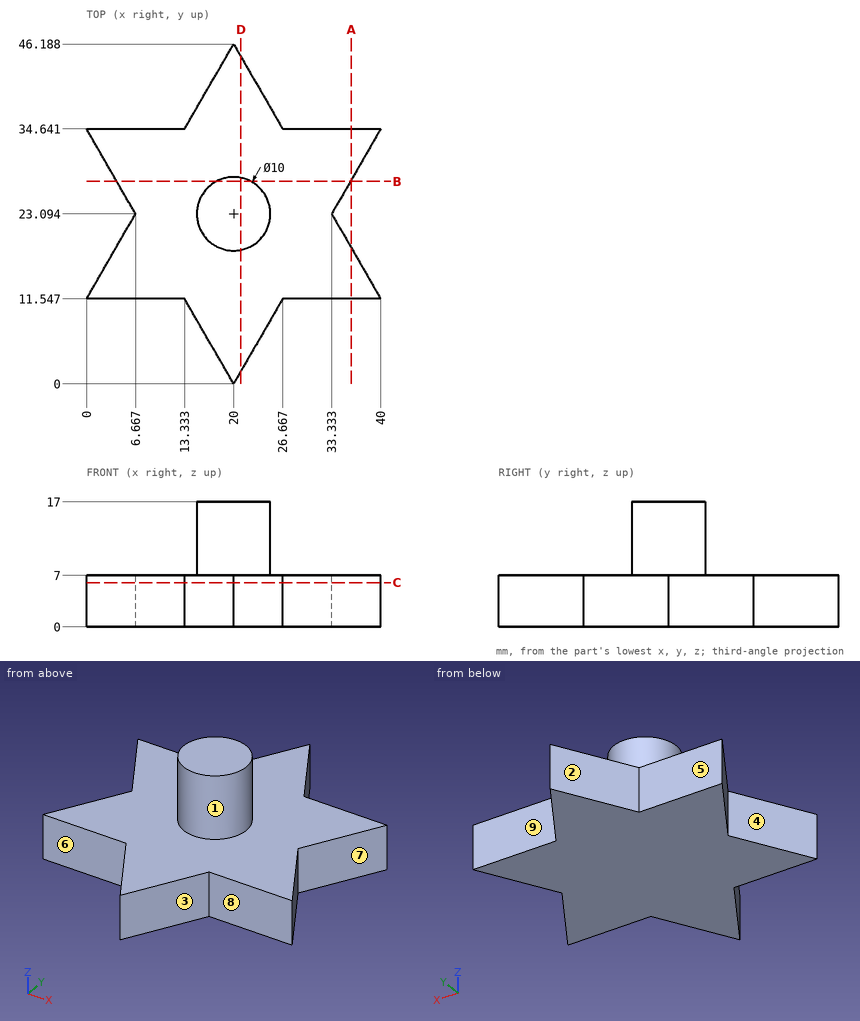
Drawing for the job (mm, zero at the part's lowest x, y, z). A direction names the side the tool comes from. Give positions to 0.01 mm unless a question says otherwise; leave off trailing zeros. Loops run counter-clockwise (first coordinate to the right, second up) from the corner with the lowest first, then second, coordinate; pieces in that order, holes last. Notation, with made-up numbers: M 7.25,-11.5 L 40.25,-11.5 A13 cw 40.25,2.5 Z; hole C 34,29 d5. An arc over 180 degrees is marked long. Use one line per item in the form item = value.
Item 1: Flat gauge pins, fed straight in: pin 1 (1.5 mm diameter, centred on x = 28.5, z = 5.5, fed in from +Y); pin 2 (1 mm diameter, centred on x = 24.5, z = 12.5, fed in from -Y) (1 decimal); pin 3 (8 mm diameter, centred on y = 19, z = 8, fed in from +X); pin 4 (8 mm diameter, centred on x = 4.5, y = 28, fed in from -Z). Where does each tip first touch, or does it go through?
Determined:
pin_1 = 34.64
pin_2 = 20.1
pin_3 = 37.93
pin_4 = 0
Item 2: Which spindle directions (+Z, -Z, +X, -X, +Y, -Y) get a long thin tool onto all of the face, cutting with end or side? Do the marked faces 5, 6, 7, 8 and 9. Say none if no direction does.
Determined:
face_5 = +Z, -Z, -X, +Y
face_6 = +Z, -Z, -X, -Y
face_7 = +Z, -Z, +X
face_8 = +Z, -Z, +X, -Y
face_9 = +Z, -Z, +X, +Y
Item 3: Slice it at A-A (x = 36). List the corners of the cut face in (y, z) (1 decimal), plus the area to 3 significant figures.
Determined:
outline = M 11.5,0 L 18.5,0 L 18.5,7 L 11.5,7 Z; M 27.7,0 L 34.6,0 L 34.6,7 L 27.7,7 Z
area = 97.0 mm2
Item 4: Slice it at D-D (x = 21). List the corners of the cut face in (y, z) (1 decimal).
Determined:
outline = M 1.7,0 L 44.5,0 L 44.5,7 L 28,7 L 28,17 L 18.2,17 L 18.2,7 L 1.7,7 Z
Item 5: Drill centre lines: probe 1 along Y at (x, z) = (32, 1.75); probe 2 along X at (y, z) = (23, 12.75); probe 3 along Z at (x, y) = (28, 17.5). Where is each one in solid material? Low to high. Write a range as from..to.
Determined:
probe_1 = 11.55..34.64
probe_2 = 15..25
probe_3 = 0..7
Item 6: Slice it at C-C (z = 6). List the corners of the cut face in (x, y), plus the area to 3 significant figures.
Determined:
outline = M 0,11.55 L 13.33,11.55 L 20,0 L 26.67,11.55 L 40,11.55 L 33.33,23.09 L 40,34.64 L 26.67,34.64 L 20,46.19 L 13.33,34.64 L 0,34.64 L 6.67,23.09 Z
area = 924 mm2
Item 7: Slice it at B-B (y = 27.5). List the corners of the cut face in (x, z).
Determined:
outline = M 4.12,0 L 35.88,0 L 35.88,7 L 22.36,7 L 22.36,17 L 17.64,17 L 17.64,7 L 4.12,7 Z
Item 8: Two-plate mould, pull along Y, no slides. Class the marked faces 1, 2, 3 and 4: pulls with the +Y half, pulls with the -Y half, needs draft (parallel to the pull), parting line crosses it, or undercut.
Determined:
face_1 = parting line crosses it
face_2 = pulls with the +Y half
face_3 = pulls with the -Y half
face_4 = undercut
